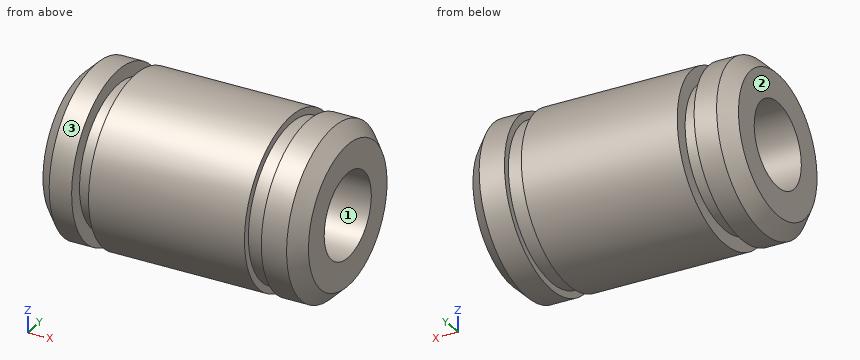
Autodesk Inventor part; units mm, degrees
ref_plane "YZ Plane" through (0, 0, 0) normal (1, 0, 0) x (0, 1, 0)
ref_plane "XZ Plane" through (0, 0, 0) normal (0, 1, 0) x (-1, 0, 0)
ref_plane "XY Plane" through (0, 0, 0) normal (0, 0, 1) x (1, 0, 0)
sketch "Sketch1" plane through (0, 0, 0) normal (0, 1, 0) x (-1, 0, 0)
  line L0 (0, 254.7362) -> (18.9, 254.7362)
  line L1 (0, 254.7362) -> (18.9, 254.7362) construction
  line L2 (18.9, 254.7362) -> (18.9, 248.7362)
  line L3 (18.9, 248.7362) -> (16.3, 248.7362)
  line L4 (16.3, 248.7362) -> (16.3, 249.7362)
  line L5 (16.3, 249.7362) -> (15.1, 249.7362)
  line L6 (15.1, 249.7362) -> (15.1, 248.7362)
  line L7 (0, 254.7362) -> (0, 248.7362)
  line L8 (0, 248.7362) -> (2.8, 248.7362)
  line L9 (2.8, 248.7362) -> (2.8, 249.2362)
  line L10 (2.8, 249.2362) -> (4, 249.2362)
  line L11 (4, 249.2362) -> (4, 248.7362)
  line L12 (4, 248.7362) -> (15.1, 248.7362)
  line L13 (18.9, 251.7362) -> (0, 251.7362)
  point P0 (0, 0)
  dimension "d0" = 18.9
  dimension "d1" = 0
  dimension "d2" = 6
  dimension "d3" = 2.6
  dimension "d4" = 1
  dimension "d5" = 1.2
  dimension "d6" = 2.8
  dimension "d7" = 1.2
  dimension "d8" = 3
revolve "Revolution1" add sketch "Sketch1" angle 360 about axis through (0, 0, 254.7362) along (-1, 0, 0) contours L13 L2 L3 L4 L5 L6 L12 L11 L10 L9 L8 L7
chamfer "Chamfer1" distance 1 angle 45 2 edges at (0, 0, 260.7362) (-18.9, 0, 260.7362)
ref_plane "Work Plane1" through (-9.45, 0, 254.7362) normal (-1, 0, 0) x (0, 0, 1)
ref_plane "Work Plane2" through (-27.2784, -18.1924, 229.4682) normal (0, -0.3925, 0.9198) x (1, 0, 0)
ref_plane "Work Plane3" through (-73.6784, -43.0389, 250.2867) normal (0, -0.9198, -0.3925) x (1, 0, 0)
properties part number "00_IGUS_Drylin_RJ4JP-01-06"
Build history of the part. All positions in model axes, mm. Face numbers are marked on the shaded views. Round coordinates to 2 decimals unless told otherwise and drop trailing zeros. Write each loop counter-clockwise with the first axis right and the second up, starting at its lowest first coordinate (ties: lowest second). Pieces come first, ordered by that corner, then holes.
1) Pin check, flat tip, straight feed: pin 1 (4 mm diameter, centred on x = -8, z = 252, fed in from +Y). Stop position of the tip, or through.
2) Band-saw the part on A-A, the plane y = 0. List the corners of the cut face in (x, z), and give its area (3 significant figures).
3) Drill centre lines: probe 1 along Z at (x, y) = (-5.75, 0); probe 2 along X at (y, z) = (1.5, 260.25); probe 3 along Y at (x, z) = (-12, 256.25). Where is each one in solid material? Low to high.
4) Band-saw the part on B-B, the plane x = -6.75. List the corners of the cut face in (y, z).
5) Mould opens along Y. For the marked faces 1, 2 and 3 say: +Y half, -Y half, draft (parallel to the pull), parting line (faces both ways), or undercut.
Ans:
1. pin 1: stops at y = 5.95
2. outline: (-18.9, 249.74) - (-17.9, 248.74) - (-16.3, 248.74) - (-16.3, 249.74) - (-15.1, 249.74) - (-15.1, 248.74) - (-4, 248.74) - (-4, 249.24) - (-2.8, 249.24) - (-2.8, 248.74) - (-1, 248.74) - (0, 249.74) - (0, 251.74) - (-18.9, 251.74) - close; (-18.9, 257.74) - (0, 257.74) - (0, 259.74) - (-1, 260.74) - (-2.8, 260.74) - (-2.8, 260.24) - (-4, 260.24) - (-4, 260.74) - (-15.1, 260.74) - (-15.1, 259.74) - (-16.3, 259.74) - (-16.3, 260.74) - (-17.9, 260.74) - (-18.9, 259.74) - close
2. area: 108 mm2
3. probe 1: z = 248.74 to 251.74, 257.74 to 260.74
3. probe 2: x = -18.19 to -16.3, -15.1 to -4, -2.8 to -0.71
3. probe 3: y = -5.81 to -2.59, 2.59 to 5.81
4. outline: circle Ø12 at (0, 254.74); hole circle Ø6 at (0, 254.74)
5. face 1: undercut
5. face 2: draft
5. face 3: parting line
